For this review, take the finished solid that the model builds, in its own axes (mm). A direction names the side the tool comes from. Coordinates: 2 decimals unless noted, no trailing zeros. Loops run counter-clockwise (first coordinate to the right, second up) from the corner with the lowest first, then second, coordinate; pieces in that order, holes last. Notation, with made-up numbers: (49.25, 0) - (55.25, 0) arc R20 cw to (55.25, 15) - close; hole circle Ø9 at (-15.5, 70). An arc over 180 degrees is marked (long way). Answer as a JSON object with one key per item and string values. Group by question number.
Item 1: We need section D-D (x = -331.5). Give the boundary of the cut face in (y, z), then the cut area to 3 significant figures.
Item 2: We need section A-A (z = 65.5). Give the boundary of the cut face in (x, y).
Item 3: We need section C-C (y = -411.5). Give the boundary of the cut face in (x, z), then the cut area to 3 significant figures.
Item 4: To check wall thickness, follow line 1 (X direction, y = -541.5, z = 88); line 2 (Y direction, x = 62, z = 32); line 3 (Z direction, x = 73.5, y = -282.5). State the ranges of each line that lie inside material, in increasing order.
Item 5: Mouldability with a two-part tool opening along Z and no side actions: class faces 4 (the flat face through (-323, -30.48, 26)), 5 (the flat face through (-398.611, -301, 26)), 6 (the flat face through (-96, -13, 50.8)) as released by +Z, released by -Z, zero draft, split by the parting line, or undercut.
Item 6: We need section B-B (z = 21). Give the boundary of the cut face in (x, y).
Item 7: Clearance check with flat-ended pins moving along their axes: pin 1 (20.5 mm diameter, centred on x = -112.5, y = -9.5, fed in from -Z); pin 2 (15 mm diameter, centred on x = -66.5, z = 23, fed in from -Y). State where each tip first meets the part, or that it passes through.
Item 8: Tool access review of faces 1 (the flat face through (-323, -316, 88.9)), 2 (the flat face through (-96, -13, 0)), 3 (the flat face through (134, -301, -50.8)): name each direction out of +Z, -Z, +X, -X, +Y, -Y from which nothing blocks a thin tool from reaching the whole face with its end or side.
from build123d import *

# Parameters (mm, degrees)
F0_W     = 127
F0_H     = 127
F0_W_2   = 304.8
F0_H_2   = 50.8
F1_DEPTH = 25.4
F2_DEPTH = 30.48
F3_DEPTH = 609.6
F4_W     = 533.4
F4_H     = 57.0844708983
F5_DEPTH = 25.4
F6_R     = 12.7
F7_W     = 533.4
F7_H     = 50.8
F8_DEPTH = 25.4
F9_R     = 12.7


with BuildPart() as f1:
    # F0 (on Front) → F1 (new body)
    with BuildSketch(Plane.XZ):
        Polygon((-398.611273554, 101.6), (-398.611273554, -50.8), (-246.211273554, -50.8), (-246.211273554, 0), (-246.211273554, 50.8), (-246.211273554, 101.6), align=None)
        with Locations((-322.411273554, 25.4)):
            Rectangle(F0_W, F0_H, mode=Mode.SUBTRACT)
        with Locations((-93.811273554, 25.4)):
            Rectangle(F0_W_2, F0_H_2)
        Polygon((58.588726446, 50.8), (58.588726446, 0), (58.588726446, -50.8), (210.988726446, -50.8), (210.988726446, 101.6), (58.588726446, 101.6), align=None)
        with Locations((134.788726446, 25.4)):
            Rectangle(F0_W, F0_H, mode=Mode.SUBTRACT)
    extrude(amount=F1_DEPTH)

    # F0 (on Front) → F2 (join)
    with BuildSketch(Plane.XZ):
        with Locations((-322.411273554, 25.4)):
            Rectangle(F0_W, F0_H)
        with Locations((134.788726446, 25.4)):
            Rectangle(F0_W, F0_H)
    extrude(amount=F2_DEPTH)

    # F0 (on Front) → F3 (join)
    with BuildSketch(Plane.XZ):
        Polygon((-398.611273554, 101.6), (-398.611273554, -50.8), (-246.211273554, -50.8), (-246.211273554, 0), (-246.211273554, 50.8), (-246.211273554, 101.6), align=None)
        with Locations((-322.411273554, 25.4)):
            Rectangle(F0_W, F0_H, mode=Mode.SUBTRACT)
        Polygon((58.588726446, 50.8), (58.588726446, 0), (58.588726446, -50.8), (210.988726446, -50.8), (210.988726446, 101.6), (58.588726446, 101.6), align=None)
        with Locations((134.788726446, 25.4)):
            Rectangle(F0_W, F0_H, mode=Mode.SUBTRACT)
    extrude(amount=F3_DEPTH)

    # F4 (on face) → F5 (cut)
    with BuildSketch(Plane.YZ.offset(-246.211273554)):
        with Locations((-317.5, 25.4)):
            Rectangle(F4_W, F4_H)
    extrude(amount=-F5_DEPTH, mode=Mode.SUBTRACT)

    # F6
    f6_edges = [f1.edges().sort_by_distance(p)[0] for p in [
        (-252.561274, -584.2, -3.142235),
        (-252.561274, -584.2, 53.942235),
        (-252.561274, -50.8, 53.942235),
        (-252.561274, -50.8, -3.142235),
    ]]
    fillet(f6_edges, radius=F6_R)

    # F7 (on face) → F8 (cut)
    with BuildSketch(Plane(origin=(58.588726446, 0, 0), x_dir=(0, -1, 0), z_dir=(-1, 0, 0))):
        with Locations((317.5, 25.4)):
            Rectangle(F7_W, F7_H)
    extrude(amount=-F8_DEPTH, mode=Mode.SUBTRACT)

    # F9
    f9_edges = [f1.edges().sort_by_distance(p)[0] for p in [
        (64.938726, -584.2, 50.8),
        (64.938726, -584.2, 0),
        (64.938726, -50.8, 0),
        (64.938726, -50.8, 50.8),
    ]]
    fillet(f9_edges, radius=F9_R)


solid = f1.part
Check sheet entries:
{
 "1": {"outline": "(-609.6, -50.8) - (0, -50.8) - (0, 101.6) - (-609.6, 101.6) - (-609.6, 88.9) - (-30.48, 88.9) - (-30.48, -38.1) - (-609.6, -38.1) - close", "area": "19,400 mm2"},
 "2": {"outline": "(-398.61, -609.6) - (-385.91, -609.6) - (-385.91, -30.48) - (-258.91, -30.48) - (-258.91, -609.6) - (-246.21, -609.6) - (-246.21, 0) - (-398.61, 0) - close; (58.59, -609.6) - (71.29, -609.6) - (71.29, -30.48) - (198.29, -30.48) - (198.29, -609.6) - (210.99, -609.6) - (210.99, 0) - (58.59, 0) - close"},
 "3": {"outline": "(-398.61, -50.8) - (-246.21, -50.8) - (-246.21, -3.14) - (-258.91, -3.14) - (-258.91, -38.1) - (-385.91, -38.1) - (-385.91, 88.9) - (-258.91, 88.9) - (-258.91, 53.94) - (-246.21, 53.94) - (-246.21, 101.6) - (-398.61, 101.6) - close; (58.59, -50.8) - (210.99, -50.8) - (210.99, 101.6) - (58.59, 101.6) - (58.59, 50.8) - (71.29, 50.8) - (71.29, 88.9) - (198.29, 88.9) - (198.29, -38.1) - (71.29, -38.1) - (71.29, 0) - (58.59, 0) - close", "area": "12,800 mm2"},
 "4": {"line 1": "x = -398.61 to -385.91, -258.91 to -246.21, 58.59 to 71.29, 198.29 to 210.99", "line 2": "y = -609.6 to -584.2, -50.8 to 0", "line 3": "z = -50.8 to -38.1, 88.9 to 101.6"},
 "5": {"face 4": "undercut", "face 5": "zero draft", "face 6": "released by +Z"},
 "6": {"outline": "(-398.61, -609.6) - (-385.91, -609.6) - (-385.91, -30.48) - (-258.91, -30.48) - (-258.91, -50.8) - (-246.21, -50.8) - (-246.21, -25.4) - (58.59, -25.4) - (58.59, -50.8) - (71.29, -50.8) - (71.29, -30.48) - (198.29, -30.48) - (198.29, -609.6) - (210.99, -609.6) - (210.99, 0) - (-398.61, 0) - close; (-258.91, -609.6) - (-246.21, -609.6) - (-246.21, -584.2) - (-258.91, -584.2) - close; (58.59, -609.6) - (71.29, -609.6) - (71.29, -584.2) - (58.59, -584.2) - close"},
 "7": {"pin 1": "stops at z = 0", "pin 2": "stops at y = -25.4"},
 "8": {"face 1": "-Y", "face 2": "-Z, +Y, -Y", "face 3": "-Z, +X, -X, +Y, -Y"}
}
